```python
from build123d import *

# Parameters (mm, degrees)
SKETCH1_W           = 203.2
SKETCH1_H           = 50.8
BOSS_EXTRUDE1_DEPTH = 12.7
CUT_EXTRUDE6_DEPTH  = 6.35


with BuildPart() as part:
    # Sketch1 → Boss-Extrude1 (new body)
    with BuildSketch(Plane(origin=(0, 0, 0), x_dir=(1, 0, 0), z_dir=(0, 1, 0))):
        with Locations((-101.6, 25.4)):
            Rectangle(SKETCH1_W, SKETCH1_H)
    extrude(amount=BOSS_EXTRUDE1_DEPTH)

    # Sketch2 → Cut-Extrude6 (cut)
    with BuildSketch(Plane(origin=(0, 12.7, 0), x_dir=(1, 0, 0), z_dir=(0, 1, 0))):
        Polygon((-176.534655494, 5.825201554), (-156.959857048, 25.4), (-176.534655494, 44.974798446), (-196.10945394, 25.4), align=None)
        Polygon((-125.734655494, 5.825201554), (-106.159857048, 25.4), (-125.734655494, 44.974798446), (-145.30945394, 25.4), align=None)
        Polygon((-74.934655494, 5.825201554), (-55.359857048, 25.4), (-74.934655494, 44.974798446), (-94.50945394, 25.4), align=None)
        Polygon((-24.134655494, 5.825201554), (-4.559857048, 25.4), (-24.134655494, 44.974798446), (-43.70945394, 25.4), align=None)
    extrude(amount=-CUT_EXTRUDE6_DEPTH, mode=Mode.SUBTRACT)


solid = part.part
```
The listing builds one solid part. Answer for the finished solid, in the listing's coordinates (mm). A direction names the side the tool comes from. Give positions to 0.01 mm unless a question says otherwise; leave off trailing zeros. Order: outer loops, then holes, each group sorted by start corner. A loop starts at its lowest first (then second) coordinate and runs counter-clockwise, first axis right, second up. Notation, with made-up numbers: (18, 25) -> (66, 25) arc R25 ccw to (66, 48) -> close; hole circle Ø8 at (-39, -15.5). An arc over 180 degrees is marked (long way). Answer as a JSON object with one key per item and string values. Group by question number.
Item 1: The part is cut by section D-D on z = -13. Write down the section's boundary in (x, y).
Item 2: The part is cut by section A-A on y = 9.75. Write down the section's boundary in (x, z).
Item 3: The part is cut by section C-C on x = -77. Write down the section's boundary in (y, z), and give its area (3 significant figures).
Item 4: Consider L1, parallel to X at y = 10.5, z = -10; L2, parallel to X at y = 11.5, z = -22.5; L3, parallel to Z at x = -16, y = 7.25. Determine where each line is inside the solid, lowest interval first. Write a range as from..to.
Item 5: Determine the mould class of faces 1 (the flat face through (-103, 6, 0)), 2 (the flat face through (-14.21, 9.57, -35.05)), 3 (the flat face through (0, 6, -25)) for opening direction X: pulls with the +X half, pulls with the -X half, needs draft (parallel to the pull), parting line crosses it, or undercut.
Item 6: The part is cut by section B-B on z = -30.5. Write down the section's boundary in (x, y), and give its area (3 significant figures).
Item 7: A flat-ended cylindrical pin translates along its axis: pin 1 (2 mm diameter, centred on y = 4, z = -30.5, fed in from +X). Find the tip coordinate at first contact, or state that the pin passes through.
Item 8: A tool of negligible diameter and unlimited length cuts with its end or side. For faces 4 (the flat face through (-84.86, 9.57, -15.75)), 5 (the flat face through (-103, 12.7, -26)), from which of +Z, -Z, +X, -X, +Y, -Y can it reach the whole face along a straight path? Write none if from no direction.
Result set:
{
 "1": {"outline": "(-203.2, 0) -> (0, 0) -> (0, 12.7) -> (-16.96, 12.7) -> (-16.96, 6.35) -> (-31.31, 6.35) -> (-31.31, 12.7) -> (-67.76, 12.7) -> (-67.76, 6.35) -> (-82.11, 6.35) -> (-82.11, 12.7) -> (-118.56, 12.7) -> (-118.56, 6.35) -> (-132.91, 6.35) -> (-132.91, 12.7) -> (-169.36, 12.7) -> (-169.36, 6.35) -> (-183.71, 6.35) -> (-183.71, 12.7) -> (-203.2, 12.7) -> close"},
 "2": {"outline": "(-203.2, -50.8) -> (0, -50.8) -> (0, 0) -> (-203.2, 0) -> close; hole (-196.11, -25.4) -> (-176.53, -44.97) -> (-156.96, -25.4) -> (-176.53, -5.83) -> close; hole (-145.31, -25.4) -> (-125.73, -44.97) -> (-106.16, -25.4) -> (-125.73, -5.83) -> close; hole (-94.51, -25.4) -> (-74.93, -44.97) -> (-55.36, -25.4) -> (-74.93, -5.83) -> close; hole (-43.71, -25.4) -> (-24.13, -44.97) -> (-4.56, -25.4) -> (-24.13, -5.83) -> close"},
 "3": {"outline": "(0, -50.8) -> (12.7, -50.8) -> (12.7, -42.91) -> (6.35, -42.91) -> (6.35, -7.89) -> (12.7, -7.89) -> (12.7, 0) -> (0, 0) -> close", "area": "423 mm²"},
 "4": {"L1": "-203.2..-180.71, -172.36..-129.91, -121.56..-79.11, -70.76..-28.31, -19.96..0", "L2": "-203.2..-193.21, -159.86..-142.41, -109.06..-91.61, -58.26..-40.81, -7.46..0", "L3": "-50.8..-36.84, -13.96..0"},
 "5": {"face 1": "needs draft", "face 2": "undercut", "face 3": "pulls with the +X half"},
 "6": {"outline": "(-203.2, 0) -> (0, 0) -> (0, 12.7) -> (-9.66, 12.7) -> (-9.66, 6.35) -> (-38.61, 6.35) -> (-38.61, 12.7) -> (-60.46, 12.7) -> (-60.46, 6.35) -> (-89.41, 6.35) -> (-89.41, 12.7) -> (-111.26, 12.7) -> (-111.26, 6.35) -> (-140.21, 6.35) -> (-140.21, 12.7) -> (-162.06, 12.7) -> (-162.06, 6.35) -> (-191.01, 6.35) -> (-191.01, 12.7) -> (-203.2, 12.7) -> close", "area": "1,850 mm²"},
 "7": {"pin 1": "x = 0"},
 "8": {"face 4": "+Y", "face 5": "+Z, -Z, +X, -X, +Y"}
}
